Geometry check sheet. Reference: drawing and pictorial views, mm from the part's lowest x, y, z. Give positions to 0.01 mm unless a question says otherwise; leave off trailing zeros. Write each loop counter-clockwise with the first axis right and the second up, starting at its lowest first coordinate (ties: lowest second). Pieces come first, ordered by that corner, then holes. Notation, with made-up numbers: (25.5, -6.5) - (54.5, -6.5) arc R18 ccw to (54.5, 21.5) - close; hole circle Ø3 at (16.5, -18.75). An arc over 180 degrees is marked (long way). Write item = value, one per line. Start each with the question number.
(1) Section check B-B, the plane y = 36.5. Enter the section's corners in (x, z), plus the area to 3 significant figures.
(2) Thickness scan on L1, parallel to Y at x = 53, z = 0.75; L2, parallel to Y at x = 75, z = 1; L3, parallel to Y at x = 26.5, z = 1.95. Record the ranges inside material, lowest first.
(3) Section check C-C, the plane x = 21. Enter the section's corners in (y, z).
(4) Section check A-A, the plane z = 1.2. Enter the section's corners in (x, y), plus the area to 3 significant figures.
(5) Depth check by flat-ended pin: pin 1 Ø1.5 at (x, z) = (32, 1) entering from -Y; pin 2 Ø1.6 at (y, z) = (31.5, 1.5) entering from -X; pin 3 Ø1 at (x, z) = (1.5, 2) entering from +Y. Enter the tip coordinate at first touch or a pass-through.
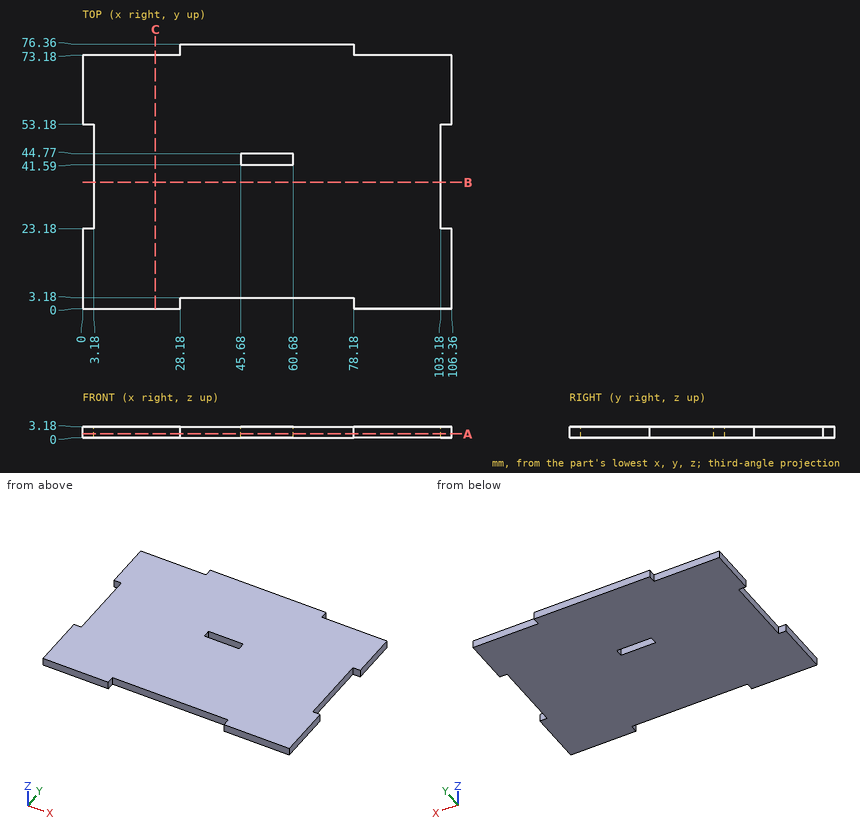
Model answer:
q1.outline = (3.18, 0) - (103.18, 0) - (103.18, 3.18) - (3.18, 3.18) - close
q1.area = 318 mm²
q2.L1 = 3.18 to 41.59, 44.77 to 76.36
q2.L2 = 3.18 to 76.36
q2.L3 = 0 to 73.18
q3.outline = (0, 0) - (73.18, 0) - (73.18, 3.18) - (0, 3.18) - close
q4.outline = (0, 0) - (28.18, 0) - (28.18, 3.18) - (78.18, 3.18) - (78.18, 0) - (106.36, 0) - (106.36, 23.18) - (103.18, 23.18) - (103.18, 53.18) - (106.36, 53.18) - (106.36, 73.18) - (78.18, 73.18) - (78.18, 76.36) - (28.18, 76.36) - (28.18, 73.18) - (0, 73.18) - (0, 53.18) - (3.18, 53.18) - (3.18, 23.18) - (0, 23.18) - close; hole (45.68, 41.59) - (60.68, 41.59) - (60.68, 44.77) - (45.68, 44.77) - close
q4.area = 7,540 mm²
q5.pin_1 = 3.18
q5.pin_2 = 3.18
q5.pin_3 = 73.18
